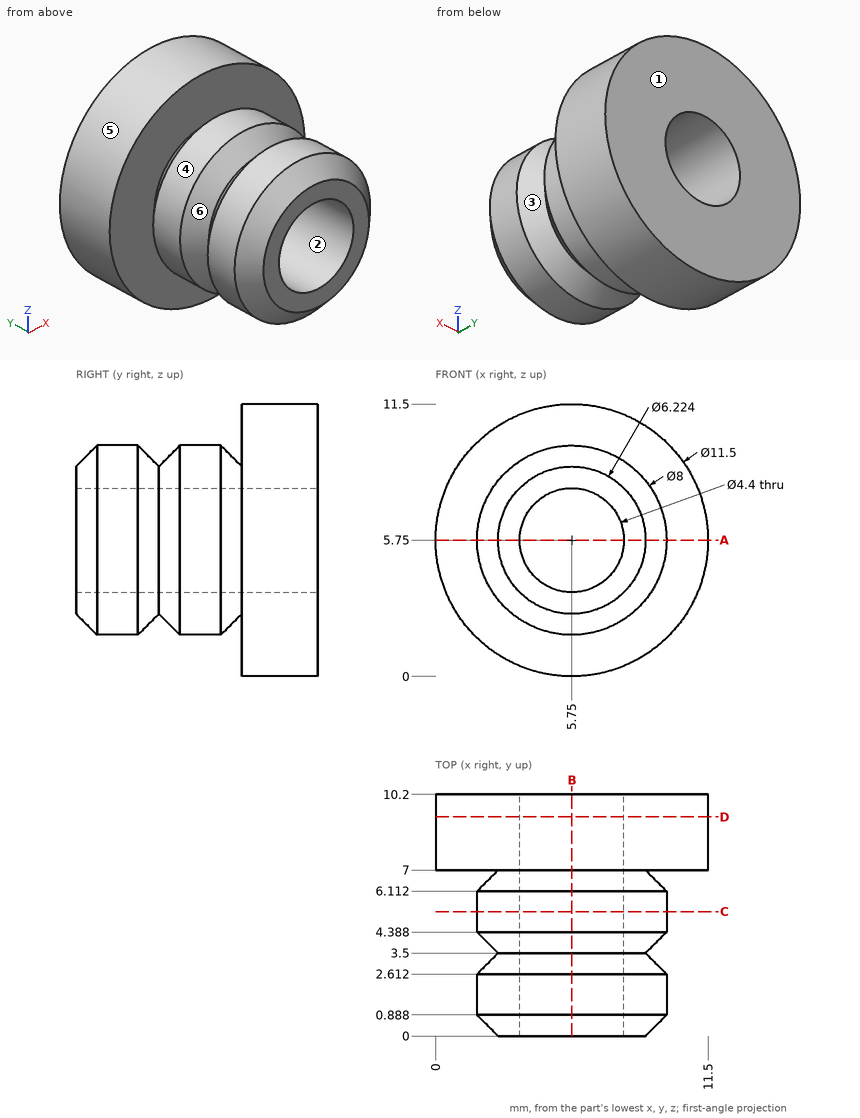
Can you work these out from the drawing? Everything is in mm from the part's minimum corner. A direction names the side the tool comes from. Round coordinates to 2 decimals unless told otherwise and drop trailing zeros. Loops run counter-clockwise (first coordinate to the right, second up) from the corner with the lowest first, then second, coordinate; pieces in that order, holes last. Notation, with made-up numbers: M 39,72.25 L 83,72.25 A17 cw 83,80.25 Z; hole C 82,-31.75 d4. An arc over 180 degrees is marked long. Answer in a Markdown table with one row per item.
1. Please list where these lines run through material, in increasing order: line 1 (X direction, y = 7.25, z = 5.75); line 2 (X direction, y = 5, z = 5.75). Write a range as from..to.
Established:
| item | result |
|---|---|
| line 1 | 0..3.55, 7.95..11.5 |
| line 2 | 1.75..3.55, 7.95..9.75 |
2. If we section it at A-A, the plane z = 5.75: Please give me the cut outline in (x, y).
Established:
| item | result |
|---|---|
| outline | M 0,7 L 2.64,7 L 1.75,6.11 L 1.75,4.39 L 2.64,3.5 L 1.75,2.61 L 1.75,0.89 L 2.64,0 L 3.55,0 L 3.55,10.2 L 0,10.2 Z; M 7.95,0 L 8.86,0 L 9.75,0.89 L 9.75,2.61 L 8.86,3.5 L 9.75,4.39 L 9.75,6.11 L 8.86,7 L 11.5,7 L 11.5,10.2 L 7.95,10.2 Z |
3. Thinking about a two-plate mould opening in X: for the marked faces 1, 2 and 3, which applies, pulls with the +X half, pulls with the -X half, needs draft (parallel to the pull), parting line crosses it, or undercut?
Established:
| item | result |
|---|---|
| face 1 | needs draft |
| face 2 | undercut |
| face 3 | parting line crosses it |
4. On a 3-axis mill with a long thin cutter (end or side, diameter ignored), from which of +Z, -Z, +X, -X, +Y, -Y can I reach the whole of each face in a straight line? I mean the marked faces 4, 5 and 6. Say none if no direction works.
Established:
| item | result |
|---|---|
| face 4 | -Y |
| face 5 | +Y, -Y |
| face 6 | none |
5. If we section it at C-C, the plane y = 5.25: Please give me the cut outline in (x, z).
Established:
| item | result |
|---|---|
| outline | C 5.75,5.75 d8; hole C 5.75,5.75 d4.4 |
6. If we section it at D-D, the plane y = 9.25: Please give me the cut outline in (x, z).
Established:
| item | result |
|---|---|
| outline | C 5.75,5.75 d11.5; hole C 5.75,5.75 d4.4 |
7. If we section it at B-B, the plane x = 5.75: Please give me the cut outline in (y, z).
Established:
| item | result |
|---|---|
| outline | M 0,2.64 L 0.89,1.75 L 2.61,1.75 L 3.5,2.64 L 4.39,1.75 L 6.11,1.75 L 7,2.64 L 7,0 L 10.2,0 L 10.2,3.55 L 0,3.55 Z; M 0,7.95 L 10.2,7.95 L 10.2,11.5 L 7,11.5 L 7,8.86 L 6.11,9.75 L 4.39,9.75 L 3.5,8.86 L 2.61,9.75 L 0.89,9.75 L 0,8.86 Z |
8. I'm going to push flat-ended pins straight in: pin 1 Ø2 at (x, y) = (6.5, 3.5) entering from -Z; pin 2 Ø5 at (y, z) = (1.5, 6) entering from -X. Where does each tip first touch, or does it pass through?
Established:
| item | result |
|---|---|
| pin 1 | z = 1.76 |
| pin 2 | x = 1.75 |
